Here's how the part is built. I have some questions about the finished solid (model axes, mm). A direction names the side the tool comes from. Round coordinates to 2 decimals unless told otherwise and drop trailing zeros. Loops run counter-clockwise (first coordinate to the right, second up) from the corner with the lowest first, then second, coordinate; pieces in that order, holes last. Notation, with made-up numbers: (28, 18) -> (87, 18) arc R23 ccw to (87, 30) -> close; hole circle Ø3 at (56, 84.5). An arc over 180 degrees is marked (long way). One line per item, written item: value. Start each with the question number.
```python
from build123d import *

# Parameters (mm, degrees)
SKETCH1_R           = 14.45
BOSS_EXTRUDE1_DEPTH = 100
FILLET1_R           = 4
SKETCH3_R           = 11
CUT_EXTRUDE1_DEPTH  = 80
FILLET2_R           = 1


with BuildPart() as part:
    # Sketch1 → Boss-Extrude1 (new body)
    with BuildSketch(Plane(origin=(0, 0, 0), x_dir=(0, 0, -1), z_dir=(1, 0, 0))):
        Circle(SKETCH1_R)
    extrude(amount=BOSS_EXTRUDE1_DEPTH)

    # Fillet1
    fillet1_edges = [part.edges().sort_by_distance(p)[0] for p in [
        (100, 0, 14.45),
    ]]
    fillet(fillet1_edges, radius=FILLET1_R)

    # Sketch3 → Cut-Extrude1 (cut)
    with BuildSketch(Plane.ZY):
        Circle(SKETCH3_R)
    extrude(amount=-CUT_EXTRUDE1_DEPTH, mode=Mode.SUBTRACT)

    # Fillet2
    fillet2_edges = [part.edges().sort_by_distance(p)[0] for p in [
        (0, 0, 14.45),
    ]]
    fillet(fillet2_edges, radius=FILLET2_R)


solid = part.part
```
Q1. If I drill on line 1 along Y through (x, z) = (32, 0); line 2 along X through (y, z) = (7.25, -3.25); line 3 along Z through (x, y) = (10.5, -1.25), over which ranges is the centre line in solid material (lowest first)?
Q2. Will these pins go through, and if not, where does the flat tip stop? P1, Ø5, axis at x = 79.5, z = -8.5, coming from the +Y side; P2, Ø10, axis at x = 31.5, z = 8.5, coming from the -Y side; P3, Ø6.5, axis at y = -5, z = 2.5, coming from the -X side.
Q3. If we mould it in two halves opening along Z, with no side actions, what happens to faces 3 (the flat face through (0, -10, 5)), 4 (the cylindrical face through (47.835, 12.184, -7.768)), 5 (the flat face through (80, 0, 0))? For each: released by +Z, released by -Z, zero draft, split by the parting line, or undercut.
Q4. I want a section at D-D on x = 82.5. Please give me the cut outline in (y, z), plus the area to 3 significant figures.
Q5. I want a section at B-B on z = 0. Please give me the cut outline in (x, y).
Q6. Which directions (+Z, -Z, +X, -X, +Y, -Y) give clear straight access to the entire face, cutting with the end or side of a thin tool? Please do faces 1 (the cylindrical face through (39.44, -10.74, -2.38)), 2 (the flat face through (100, 0, 0)).
Q7. I want a section at A-A on x = 23. Please give me the cut outline in (y, z), plus the area to 3 significant figures.
Answers below:
1. line 1: y = -14.45 to -11, 11 to 14.45
1. line 2: x = 80 to 100
1. line 3: z = -14.4 to -10.93, 10.93 to 14.4
2. P1: stops at y = 13.15
2. P2: stops at y = -14.02
2. P3: stops at x = 80
3. face 3: zero draft
3. face 4: split by the parting line
3. face 5: undercut
4. outline: circle Ø28.9 at (0, 0)
4. area: 656 mm^2
5. outline: (0, -13.45) arc R1 ccw to (1, -14.45) -> (96, -14.45) arc R4 ccw to (100, -10.45) -> (100, 10.45) arc R4 ccw to (96, 14.45) -> (1, 14.45) arc R1 ccw to (0, 13.45) -> (0, 11) -> (80, 11) -> (80, -11) -> (0, -11) -> close
6. face 1: -X
6. face 2: +Z, -Z, +X, +Y, -Y
7. outline: circle Ø28.9 at (0, 0); hole circle Ø22 at (0, 0)
7. area: 276 mm^2
